Design review of the part built by this model. Coordinates are the model's own, in mm. A direction names the side the tool comes from. Round coordinates to 2 decimals unless told otherwise and drop trailing zeros. Order: outer loops, then holes, each group sorted by start corner. A loop starts at its lowest first (then second) coordinate and runs counter-clockwise, first axis right, second up. Notation, with made-up numbers: (34, 46.25) - (80, 46.25) arc R8 ccw to (80, 51.25) - close; hole circle Ø11 at (64, 53.5). An arc over 180 degrees is marked (long way). Use CSV: the item, a comma, the result in double quotes.
from build123d import *

# Parameters (mm, degrees)
F0_W     = 41.275
F0_H     = 50.8
F0_R     = 1.5875
F1_DEPTH = 3.175
F2_W     = 41.275
F2_H     = 3.175
F3_DEPTH = 12.7
F5_W     = 25.4
F5_H     = 28.575
F6_DEPTH = 3.175
F4_R     = 1.143
F7_DEPTH = 25.4
F8_R     = 5.08
F9_R     = 5.08


with BuildPart() as f1:
    # F0 (on Front) → F1 (new body)
    with BuildSketch(Plane.XZ):
        with Locations((-1.74602, 12.366909)):
            Rectangle(F0_W, F0_H)
        with Locations((-17.62102, -6.683091)):
            Circle(F0_R, mode=Mode.SUBTRACT)
        with Locations((14.12898, -6.683091)):
            Circle(F0_R, mode=Mode.SUBTRACT)
    extrude(amount=F1_DEPTH)

    # F2 (on face) → F3 (join)
    with BuildSketch(Plane.XZ.offset(3.175)):
        with Locations((-1.74602, 36.179409)):
            Rectangle(F2_W, F2_H)
    extrude(amount=F3_DEPTH)

    # F5 (on face) → F6 (cut)
    with BuildSketch(Plane.XZ.offset(3.175)):
        with Locations((-1.74602, 17.129409)):
            Rectangle(F5_W, F5_H)
    extrude(amount=-F6_DEPTH, mode=Mode.SUBTRACT)

    # F4 (on face) → F7 (cut)
    with BuildSketch(Plane.XY.offset(37.766909)):
        with Locations((-6.50852, -9.525)):
            Circle(F4_R)
    extrude(amount=-F7_DEPTH, mode=Mode.SUBTRACT)

    # F8
    f8_edges = [f1.edges().sort_by_distance(p)[0] for p in [
        (-22.38352, -15.875, 36.179409),
    ]]
    fillet(f8_edges, radius=F8_R)

    # F9
    f9_edges = [f1.edges().sort_by_distance(p)[0] for p in [
        (18.89148, -15.875, 36.179409),
    ]]
    fillet(f9_edges, radius=F9_R)


solid = f1.part
1) To check wall thickness, follow L1, parallel to Z at x = 14, y = -3; L2, parallel to Y at x = -19, z = 14 (3 decimals); L3, parallel to Z at x = -14, y = -13.5. State the ranges of each line that lie inside material, in increasing order. Write a range as from..to.
Data:
L1,"z = -13.03..-8.27, -5.1..37.77"
L2,"y = -3.175..0"
L3,"z = 34.59..37.77"
2) We need section B-B (z = 26.5). Give the boundary of the cut face in (x, y) (3 decimals), then the cut area to 3 significant figures.
Data:
outline,"(-22.384, -3.175) - (-14.446, -3.175) - (-14.446, 0) - (-22.384, 0) - close; (10.954, -3.175) - (18.891, -3.175) - (18.891, 0) - (10.954, 0) - close"
area,"50.4 mm2"
3) Insertion check: pin 1 Ø3.5 at (x, z) = (14.13, -6.68) entering from -Y (3 decimals); pin 2 Ø6.5 at (x, y) = (-2.5, -8) entering from -Z. Each pin has a flat end and moves straight along its axis. Give the tip position at first contact, or say it passes through.
Data:
pin 1,"stops at y = -3.175"
pin 2,"stops at z = 34.59"
4) We need section D-D (y = -1.75). Give the boundary of the cut face in (x, z) (1 decimal), then the cut area to 3 significant figures.
Data:
outline,"(-22.4, -13) - (18.9, -13) - (18.9, 37.8) - (-22.4, 37.8) - close; hole circle Ø3.2 at (-17.6, -6.7); hole (-14.4, 2.8) - (11, 2.8) - (11, 31.4) - (-14.4, 31.4) - close; hole circle Ø3.2 at (14.1, -6.7)"
area,"1,360 mm2"
5) We need section A-A (x = -2). Give the boundary of the cut face in (y, z) (3 decimals).
Data:
outline,"(-15.875, 34.592) - (-3.175, 34.592) - (-3.175, 31.417) - (0, 31.417) - (0, 37.767) - (-15.875, 37.767) - close; (-3.175, -13.033) - (0, -13.033) - (0, 2.842) - (-3.175, 2.842) - close"
6) For faces 4 (the face through (-2, 0, 1)), 5 (the face through (-2, -2, 2.842)), 6 (the face through (-2, -9, 34.592)), list the 3-axis set-ups (+Z, -Z, +X, -X, +Y, -Y) from which the entire face can be reached by the end or side of a thin tool; tool diameter is ignored.
Data:
face 4,"+Z, -Z, +X, -X, +Y"
face 5,"+Y, -Y"
face 6,"-Z, +X, -X, -Y"
7) The part is to be moulded in two halves that separate along X. For faces 1 (the face through (17.36, -14.43, 36.2)), 2 (the face through (15.595, -1.565, -7.291)), 3 (the face through (-22.384, -2, 16)), say which applies: +X half, -X half, draft (parallel to the pull), parting line (faces both ways), or undercut.
Data:
face 1,"+X half"
face 2,"undercut"
face 3,"-X half"
8) We need section C-C (y = -7.5). Give the boundary of the cut face in (x, z).
Data:
outline,"(-22.38, 34.59) - (18.89, 34.59) - (18.89, 37.77) - (-22.38, 37.77) - close"
